The listing builds one solid part. Answer for the finished solid, in the listing's coordinates (mm). Face numbers are marked on the shaded views. A direction names the side the tool comes from. Coordinates: 2 decimals unless noted, no trailing zeros. Order: outer loops, then holes, each group sorted by start corner. A loop starts at its lowest first (then second) coordinate and runs counter-clockwise, first axis right, second up. Notation, with made-up numbers: (57.5, 59.5) -> (88.5, 59.5) arc R16 ccw to (88.5, 86.5) -> close; hole circle Ø7 at (-19.75, 18.5). An arc over 180 degrees is marked (long way). Return JSON: item names as keys, results as strings.
```python
from build123d import *

# Parameters (mm, degrees)
PAD_DEPTH           = 5
PAD001_DEPTH        = 20
PAD002_DEPTH        = 50
LINEARPATTERN_COUNT = 8
LINEARPATTERN_PITCH = 12
SKETCH003_R         = 1.6
HOLE_DEPTH          = 20
HOLE_TIPS_R         = 1.6
CHAMFER_SIZE        = 4
CHAMFER001_SIZE     = 1
FILLET_R            = 2


with BuildPart() as obj1:
    # Sketch → Pad (new body)
    with BuildSketch(Plane.XZ):
        Polygon((-50, -50), (-50, 50), (0, 50), (0, 75), (-60, 75), (-75, 60), (-75, -60), (-60, -75), (0, -75), (0, -50), align=None)
    extrude(amount=PAD_DEPTH)

    # Sketch001 → Pad001 (join)
    with BuildSketch(Plane.XZ):
        Polygon((0, 56), (-56, 56), (-56, 0), (-56, -56), (0, -56), (0, -50), (-50, -50), (-50, 0), (-50, 50), (0, 50), align=None)
    extrude(amount=-PAD001_DEPTH)

    # Sketch002 (on Face5 of Pad001) → Pad002 (join)
    with BuildSketch(Plane(origin=(-50, 0, 0), x_dir=(0, 0, 1), z_dir=(1, 0, 0))):
        Polygon((39, 5), (47, -0.839889), (47, -2.664855), (36.5, 5), align=None)
    pad002 = extrude(amount=PAD002_DEPTH)

    # LinearPattern: Pad002 ×8
    with Locations(*[(0, 0, -i * LINEARPATTERN_PITCH) for i in range(1, LINEARPATTERN_COUNT)]):
        add(pad002)

    # Sketch003 (on Face22 of LinearPattern) → Hole (cut)
    with BuildSketch(Plane(origin=(0, 20, 0), x_dir=(1, 0, 0), z_dir=(0, 1, 0))):
        with Locations((-25, 53)):
            Circle(SKETCH003_R)
        with Locations((-53, 0)):
            Circle(SKETCH003_R)
        with Locations((-25, -53)):
            Circle(SKETCH003_R)
    extrude(amount=-HOLE_DEPTH, mode=Mode.SUBTRACT)

    # Hole tips → Hole tip 1 section 0
    with BuildSketch(Plane(origin=(0, 0, 0), x_dir=(1, 0, 0), z_dir=(0, 1, 0)), mode=Mode.PRIVATE) as hole_tip_1_s0:
        with Locations((-25, 53)):
            Circle(HOLE_TIPS_R)
    loft([hole_tip_1_s0.sketch, Vertex(-25, -0.961377, -53)], mode=Mode.SUBTRACT)

    # Hole tips → Hole tip 2 section 0
    with BuildSketch(Plane(origin=(0, 0, 0), x_dir=(1, 0, 0), z_dir=(0, 1, 0)), mode=Mode.PRIVATE) as hole_tip_2_s0:
        with Locations((-53, 0)):
            Circle(HOLE_TIPS_R)
    loft([hole_tip_2_s0.sketch, Vertex(-53, -0.961377, 0)], mode=Mode.SUBTRACT)

    # Hole tips → Hole tip 3 section 0
    with BuildSketch(Plane(origin=(0, 0, 0), x_dir=(1, 0, 0), z_dir=(0, 1, 0)), mode=Mode.PRIVATE) as hole_tip_3_s0:
        with Locations((-25, -53)):
            Circle(HOLE_TIPS_R)
    loft([hole_tip_3_s0.sketch, Vertex(-25, -0.961377, 53)], mode=Mode.SUBTRACT)

    # Chamfer
    chamfer_edges = [obj1.edges().sort_by_distance(p)[0] for p in [
        (-30, -5, 75),
        (-67.5, -5, 67.5),
        (-75, -5, 0),
        (-67.5, -5, -67.5),
        (-30, -5, -75),
    ]]
    chamfer(chamfer_edges, length=CHAMFER_SIZE)

    # Chamfer001
    chamfer001_edges = [obj1.edges().sort_by_distance(p)[0] for p in [
        (-23.4, 20, 53),
        (-51.4, 20, 0),
        (-23.4, 20, -53),
    ]]
    chamfer(chamfer001_edges, length=CHAMFER001_SIZE)

    # Fillet
    fillet_edges = [obj1.edges().sort_by_distance(p)[0] for p in [
        (-25, -5, 50),
        (-50, -5, 44.5),
        (-50, -5, 31.75),
        (-50, -5, 19.75),
        (-50, -5, 7.75),
        (-50, -5, -4.25),
        (-50, -5, -16.25),
        (-50, -5, -28.25),
        (-50, -5, -40.25),
        (-50, -5, -48.75),
        (-25, -5, -50),
    ]]
    fillet(fillet_edges, radius=FILLET_R)


with BuildPart() as part_mirroring:
    # Part__Mirroring: instance of obj1
    add(obj1.part.mirror(Plane(origin=(0, 0, 0), x_dir=(0, -1, 0), z_dir=(1, 0, 0))))


solid = part_mirroring.part
```
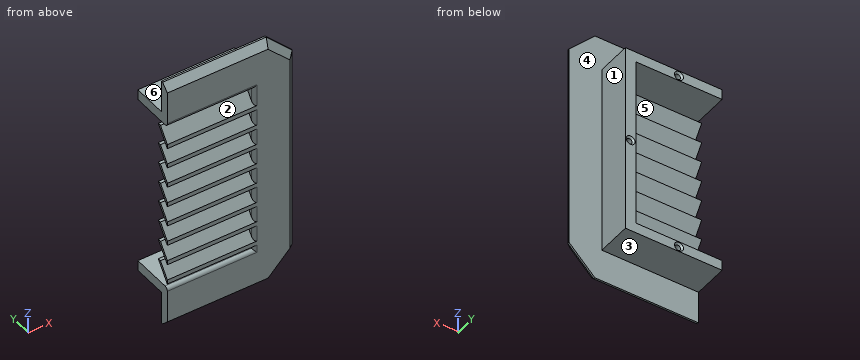
Item 1: The part is cut by section B-B on z = 9. Determine the outline of the cut face in (x, y).
Answer list:
{"outline": "(0, -0.62) -> (50, -0.62) -> (50, -3) arc R2 ccw to (52, -5) -> (71, -5) -> (75, -1) -> (75, 0) -> (56, 0) -> (56, 20) -> (50, 20) -> (50, 1.2) -> (0, 1.2) -> close"}
Item 2: Which of the six approach directions +Z, -Z, +X, -X, +Y, -Y give full straight-line access (tool end or side, diameter ignored) to the marked faces 1, 2 and 3?
Answer list:
{"face 1": "+Z, -Z, +X, +Y", "face 2": "-X, -Y", "face 3": "-Z, +X, -X, +Y"}
Item 3: Determine the mould class of the marked faces 4, 5 and 6 for opening direction Z: pulls with the +Z half, pulls with the -Z half, needs draft (parallel to the pull), parting line crosses it, or undercut.
Answer list:
{"face 4": "needs draft", "face 5": "undercut", "face 6": "pulls with the +Z half"}
Item 4: The part is cut by section D-D on z = 62.5. Determine the outline of the cut face in (x, y).
Answer list:
{"outline": "(0, -5) -> (66.84, -5) -> (72.5, -1) -> (72.5, 0) -> (0, 0) -> close"}
Item 5: The part is cut by section C-C on x = 42.5. Count the separate pieces of the cut face and the enclosed holes in it, plus the area to 3 significant figures.
Answer list:
{"separate pieces": "10", "enclosed holes": "0", "area": "607 mm2"}
Item 6: The part is cut by section A-A on y = 7.25. Determine the outline of the cut face in (x, z).
Answer list:
{"outline": "(0, -56) -> (56, -56) -> (56, 56) -> (0, 56) -> (0, 50) -> (50, 50) -> (50, -50) -> (0, -50) -> close; hole circle Ø3.2 at (25, -53); hole circle Ø3.2 at (25, 53); hole circle Ø3.2 at (53, 0)"}
Item 7: Find the intervals of material crossed by probe 1 along Z at (x, y) = (25, 4); probe 2 along Z at (x, y) = (24.5, 17.25); probe 3 along X at (y, z) = (15, 0), in increasing order.
Answer list:
{"probe 1": "-56 to -54.6, -51.4 to -50, 50 to 51.4, 54.6 to 56", "probe 2": "-56 to -54.52, -51.48 to -50, 50 to 51.48, 54.52 to 56", "probe 3": "50 to 51.4, 54.6 to 56"}
Item 8: Flat-ended cylindrical pins translate along their axes: pin 1 (6 mm diameter, centred on x = 20, y = 15, fed in from +Z); pin 2 (4 mm diameter, centred on y = 15.5, z = 57.5, fed in from +X); pin 3 (1.9 mm diameter, centred on x = 25, z = 53, fed in from +Y). Find the tip coordinate at first contact, or state that the pin passes through.
Answer list:
{"pin 1": "z = 56", "pin 2": "x = 56", "pin 3": "y = -0.39"}
